CAD build for the part. Positions are in the model's coordinates, mm. Face numbers are marked on the shaded views. A direction names the side the tool comes from. Coordinates: 2 decimals unless noted, no trailing zeros. Loops run counter-clockwise (first coordinate to the right, second up) from the corner with the lowest first, then second, coordinate; pieces in that order, holes last. Notation, with made-up numbers: (43.25, -28) -> (92.25, -28) arc R18 cw to (92.25, 1) -> close; hole circle Ø2 at (24, 70). An arc over 180 degrees is marked (long way). Write item = value, one per line. Start each with the question number.
(1) Tool access for the marked faces 5 and 6: list every direction of +Z, -Z, +X, -X, +Y, -Y with a clear straight run to the whole face (end or side of a thin tool).
(2) Band-saw the part on B-B (y = 5.6). Write the cut outline in (x, z).
(3) Band-saw the part on D-D (z = 3). Write the cut outline in (x, y).
(4) Band-saw the part on A-A (x = -5.1). Write the cut outline in (y, z).
(5) Band-saw the part on C-C (x = 8). Write the cut outline in (y, z), and give its area (3 significant figures).
(6) Drill centre lines: line 1 (Y direction, x = -7.5, z = 6); line 2 (Y direction, x = -4.25, z = 2); line 3 (X direction, y = 2, z = 6.5). Where is each one in solid material? Low to high. Write a range as from..to.
(7) Flat gauge pin, fed straight in: P1, Ø3.5, axis at x = -5.1, y = 5.6, coming from the -Z side. Where does the tip first touch, or does it go through?
(8) Pull direction X, two halves, no side cores. Call the marked faces 1, 2, 3 and 4: +X half, -X half, draft (parallel to the pull), parting line (faces both ways), or undercut.
```python
from build123d import *

# Parameters (mm, degrees)
F0_W       = 22
F0_H       = 2
F0_R       = 1.5
F1_DEPTH   = 4.7
F2_DEPTH   = 8.7
F3_R       = 1.5
F4_DEPTH   = 4.701
F6_SIZE2   = 1
F6_SIZE    = 0.5
F6_2_SIZE2 = 1
F6_2_SIZE  = 0.5
F6_3_SIZE2 = 1
F6_3_SIZE  = 0.5
F7_R       = 3
F8_R       = 1.99999
F5_R       = 1.15
F9_DEPTH   = 26.0010001


# Not quite as in the source:
# - a fillet or chamfer is up to 0.001 mm smaller than in the source, because OpenCascade refuses the exact size


with BuildPart() as f1:
    # F0 (on Top) → F1 (new body)
    with BuildSketch(Plane.XY):
        with Locations((0, 12.5)):
            Rectangle(F0_W, F0_H)
        Polygon((-11, -12.5), (-11, 11.5), (-11, 13.5), (-13, 13.5), (-13, -14.5), (-11, -14.5), align=None)
        Polygon((11, 13.5), (11, 11.5), (11, -12.5), (11, -14.5), (13, -14.5), (13, 13.5), align=None)
        Polygon((4, -12.5), (-11, -12.5), (-11, -14.5), (11, -14.5), (11, -12.5), (6.7, -12.5), align=None)
        Polygon((11, 11.5), (-11, 11.5), (-11, -12.5), (4, -12.5), (4, 0), (6.7, 0), (6.7, -12.5), (11, -12.5), align=None)
        with Locations((-5.1, 5.6)):
            Circle(F0_R, mode=Mode.SUBTRACT)
    extrude(amount=F1_DEPTH)

    # F0 (on Top) → F2 (join)
    with BuildSketch(Plane.XY):
        Polygon((11, 13.5), (11, 11.5), (11, -12.5), (11, -14.5), (13, -14.5), (13, 13.5), align=None)
        Polygon((4, -12.5), (-11, -12.5), (-11, -14.5), (11, -14.5), (11, -12.5), (6.7, -12.5), align=None)
        Polygon((-11, -12.5), (-11, 11.5), (-11, 13.5), (-13, 13.5), (-13, -14.5), (-11, -14.5), align=None)
        with Locations((0, 12.5)):
            Rectangle(F0_W, F0_H)
    extrude(amount=F2_DEPTH)

    # F3 (on face) → F4 (cut, through all)
    with BuildSketch(Plane.XY.offset(4.7)):
        with Locations((-5.1, 5.6)):
            Circle(F3_R)
    extrude(amount=-F4_DEPTH, mode=Mode.SUBTRACT)

    # F6
    f6_edges = [f1.edges().sort_by_distance(p)[0] for p in [
        (0, 11.5, 8.7),
        (11, -0.5, 8.7),
        (-11, -0.5, 8.7),
        (0, -12.5, 8.7),
    ]]
    f6_side = f1.faces().sort_by_distance((11.382099, -0.5, 8.7))[0]
    chamfer(f6_edges, length=F6_SIZE, length2=F6_SIZE2, reference=f6_side)

    # F6#2
    f6_2_edges = [f1.edges().sort_by_distance(p)[0] for p in [
        (-6.6, 5.6, 0),
    ]]
    f6_2_side = f1.faces().sort_by_distance((-0.210298, -0.280343, 0))[0]
    chamfer(f6_2_edges, length=F6_2_SIZE, length2=F6_2_SIZE2, reference=f6_2_side)

    # F6#3
    f6_3_edges = [f1.edges().sort_by_distance(p)[0] for p in [
        (5.35, 0, 4.7),
        (4, -6.25, 4.7),
    ]]
    f6_3_side = f1.faces().sort_by_distance((-0.29663, -0.190169, 4.7))[0]
    chamfer(f6_3_edges, length=F6_3_SIZE, length2=F6_3_SIZE2, reference=f6_3_side)

    # F7
    f7_edges = [f1.edges().sort_by_distance(p)[0] for p in [
        (-13, -14.5, 4.35),
        (13, -14.5, 4.35),
        (-13, 13.5, 4.35),
        (13, 13.5, 4.35),
    ]]
    fillet(f7_edges, radius=F7_R)

    # F8 (radius 2 in the source; OpenCascade refuses exactly that, so slightly less here)
    f8_edges = [f1.edges().sort_by_distance(p)[0] for p in [
        (13, -0.5, 0),
        (12.12132, -13.62132, 0),
        (0, -14.5, 0),
        (-12.12132, -13.62132, 0),
        (12.12132, 12.62132, 0),
        (0, 13.5, 0),
        (-12.12132, 12.62132, 0),
        (-13, -0.5, 0),
    ]]
    fillet(f8_edges, radius=F8_R)

    # F5 (on face) → F9 (cut, through all)
    with BuildSketch(Plane.YZ.offset(13)):
        with Locations((-6.6, 2.3)):
            Circle(F5_R)
    extrude(amount=-F9_DEPTH, mode=Mode.SUBTRACT)


solid = f1.part
```
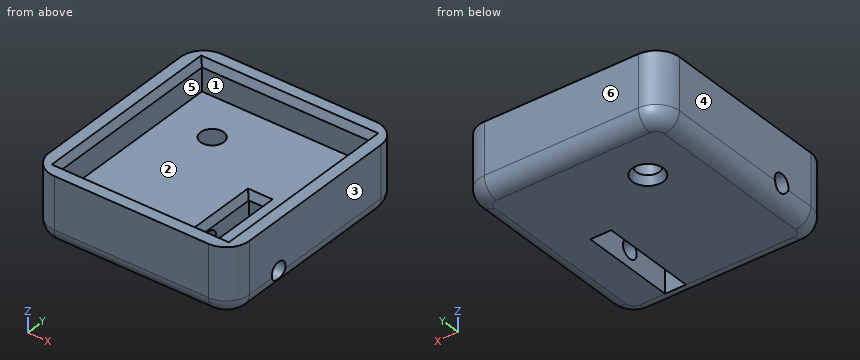
Findings below:
q1.face_5 = +Z
q1.face_6 = +Z, -Z, +X, -X, +Y
q2.outline = (-13, 2) arc R2 ccw to (-11, 0) -> (-7.1, 0) -> (-6.6, 1) -> (-6.6, 4.7) -> (-11, 4.7) -> (-11, 7.7) -> (-11.5, 8.7) -> (-13, 8.7) -> close; (-3.6, 1) -> (-3.1, 0) -> (11, 0) arc R2 ccw to (13, 2) -> (13, 8.7) -> (11.5, 8.7) -> (11, 7.7) -> (11, 4.7) -> (-3.6, 4.7) -> close
q3.outline = (-13, -11.5) arc R3 ccw to (-10, -14.5) -> (10, -14.5) arc R3 ccw to (13, -11.5) -> (13, -7.51) -> (6.7, -7.51) -> (6.7, -12.5) -> (4, -12.5) -> (4, -7.51) -> (-13, -7.51) -> close; (-13, -5.69) -> (4, -5.69) -> (4, 0) -> (6.7, 0) -> (6.7, -5.69) -> (13, -5.69) -> (13, 10.5) arc R3 ccw to (10, 13.5) -> (-10, 13.5) arc R3 ccw to (-13, 10.5) -> close; hole circle Ø3 at (-5.1, 5.6)
q4.outline = (-14.5, 2) arc R2 ccw to (-12.5, 0) -> (3.6, 0) -> (4.1, 1) -> (4.1, 4.7) -> (-12.5, 4.7) -> (-12.5, 7.7) -> (-13, 8.7) -> (-14.5, 8.7) -> close; (7.1, 1) -> (7.6, 0) -> (11.5, 0) arc R2 ccw to (13.5, 2) -> (13.5, 8.7) -> (12, 8.7) -> (11.5, 7.7) -> (11.5, 4.7) -> (7.1, 4.7) -> close; hole circle Ø2.3 at (-6.6, 2.3)
q5.outline = (-14.5, 2) arc R2 ccw to (-12.5, 0) -> (11.5, 0) arc R2 ccw to (13.5, 2) -> (13.5, 8.7) -> (12, 8.7) -> (11.5, 7.7) -> (11.5, 4.7) -> (-12.5, 4.7) -> (-12.5, 7.7) -> (-13, 8.7) -> (-14.5, 8.7) -> close; hole circle Ø2.3 at (-6.6, 2.3)
q5.area = 141 mm²
q6.line_1 = -14.5..-12.5, 11.5..13.5
q6.line_2 = -14.5..-7.71, -5.49..4.36, 6.84..13.5
q6.line_3 = -13..-11, 11..13
q7.P1 = 0.5
q8.face_1 = undercut
q8.face_2 = undercut
q8.face_3 = +X half
q8.face_4 = -X half
